The figure shows three views and two pictorial views of one solid part (mm, origin at its lowest corner). Answer the questions. A direction names the side the tool comes from. Give positions to 0.01 mm unless a question says otherwise; leave off trailing zeros. Write item = value, one per line.
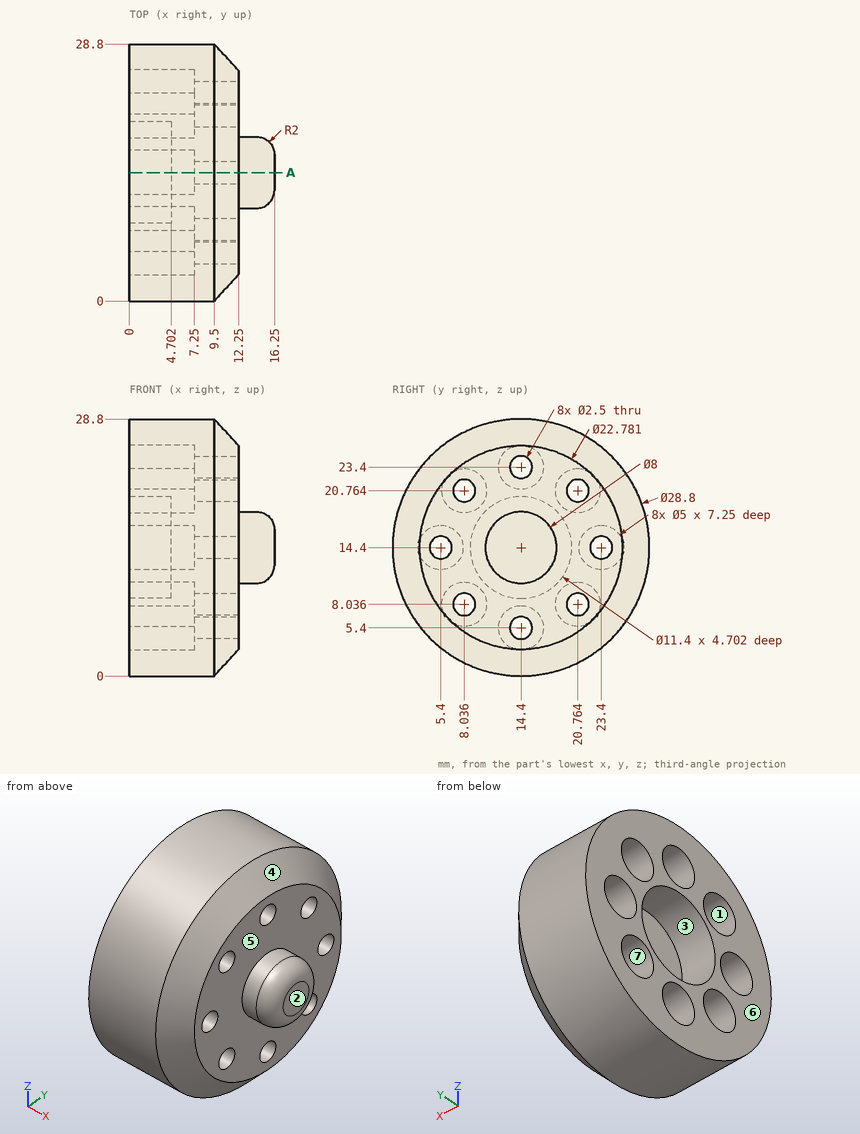
1. Determine the mould class of the marked faces 1, 2, 3 and 4 for opening direction Z: +Z half, -Z half, draft (parallel to the pull), parting line (faces both ways), or undercut.
Recorded:
face_1 = undercut
face_2 = draft
face_3 = undercut
face_4 = parting line
2. Flat-ended cylindrical pins translate along their axes: pin 1 (5 mm diameter, centred on y = 4.5, z = 12, fed in from +X); pin 2 (6 mm diameter, centred on y = 18, z = 7.5, fed in from -X); pin 3 (4 mm diameter, centred on y = 14.4, z = 23.4, fed in from -X); pin 4 (3.5 mm diameter, centred on y = 16, z = 16.5, fed in from -X). Find the tip coordinate at first contact, or state that the pin passes through.
Recorded:
pin_1 = 12.25
pin_2 = 0
pin_3 = 7.25
pin_4 = 4.7
3. Straight lines are drawn through the part: L1, parallel to Y at x = 4, z = 12.25 (1 decimal); L2, parallel to X at y = 18.75, z = 8.5; L3, parallel to X at y = 5, z = 8.75. For each, find the intervals that lie inside material, in ascending order. Write a range as [from, to].
Recorded:
L1 = [0.2, 4.1], [6.7, 9.1], [19.7, 22.1], [24.7, 28.6]
L2 = [7.25, 12.25]
L3 = [0, 12.25]
4. Section A-A (y = 14.4) is taken. Count the separate pieces of the cut face and the enclosed holes in it, and give its area (3 significant figures).
Recorded:
separate_pieces = 3
enclosed_holes = 0
area = 224 mm^2
5. For the marked faces 5, 6 and 7, determine the directions among +Z, -Z, +X, -X, +Y, -Y from which every point of the face is accessible in a straight line to the end or side of a thin tool.
Recorded:
face_5 = +X
face_6 = +Z, -Z, -X, +Y, -Y
face_7 = -X
